Check sheet for the modelled part. Datum: model origin and axes. Units: mm. Coordinates: 2 decimals unless noted, no trailing zeros. Loops run counter-clockwise (first coordinate to the right, second up) from the corner with the lowest first, then second, coordinate; pieces in that order, holes last. Notation, with made-up numbers: (21, 77) - (32, 77) arc R23 ccw to (32, 87) - close; hole circle Ø11 at (12, 67.5). An arc over 180 degrees is marked (long way). Use a Markdown table: item, result. Add a question column.
1) Go/stop test with flat-tipped pins: P1, Ø3, axis at x = 56.5, z = -72.5, coming from the -Y side; P2, Ø9.5, axis at x = -42.43, z = 42.43, coming from the -Y side; P3, Ø3.5, axis at x = -56.5, z = -57.5, coming from the +Y side. Record where each tip stops, or that it passes through.
2) Thickness scan on line 1 (Z direction, x = -72.5, y = 0.25); line 2 (X direction, y = 0.35, z = 72.5); line 3 (Z direction, x = -42.5, y = 0.95). Record the ranges inside material, lowest first.
3) Sectioned sample at A-A, the plane x = -12. Enter the section's corners in (y, z).
4) Sectioned sample at B-B, the plane y = 2.3. State how many separate pieces and enclosed holes the cut face has, then the cut area to 3 significant figures.
5) Sectioned sample at C-C, the plane x = 44.5. Enter the section's corners in (y, z), then the cut area to 3 significant figures.
6) Draft check along Z on faces 1 (the cylindrical face through (-55.984, 1.479, -0.527)), 2 (the flat face through (-1, 0, -1)). Enter one of: pulls with the +Z half, pulls with the -Z half, needs draft (parallel to the pull), parting line crosses it, or undercut.
from build123d import *

# Parameters (mm, degrees)
SKETCH_1_W      = 155
SKETCH_1_H      = 154
SKETCH_1_R      = 1.55
SKETCH_1_R_2    = 2.05
SKETCH_1_R_3    = 4.05
EXTRUDE_1_DEPTH = 3
FILLET_1_R      = 1.5
CHAMFER_1_SIZE  = 1.5
CHAMFER_1_SIZE2 = 2.598076211


with BuildPart() as part:
    # 草图1 → 凸台-拉伸1 (new body)
    with BuildSketch(Plane(origin=(0, 0, 0), x_dir=(1, 0, 0), z_dir=(0, 1, 0))):
        Rectangle(SKETCH_1_W, SKETCH_1_H)
        with Locations(Location((56.5, 72.5, 0), (0, 0, 270))):
            Circle(SKETCH_1_R, mode=Mode.SUBTRACT)
        with Locations(Location((72.5, 72.5, 0), (0, 0, 270))):
            Circle(SKETCH_1_R, mode=Mode.SUBTRACT)
        with Locations(Location((72.5, 57.5, 0), (0, 0, 90))):
            Circle(SKETCH_1_R, mode=Mode.SUBTRACT)
        with Locations(Location((56.5, 57.5, 0), (0, 0, 90))):
            Circle(SKETCH_1_R, mode=Mode.SUBTRACT)
        with Locations(Location((-56.5, 57.5, 0), (0, 0, 270))):
            Circle(SKETCH_1_R, mode=Mode.SUBTRACT)
        with Locations(Location((-72.5, 57.5, 0), (0, 0, 270))):
            Circle(SKETCH_1_R, mode=Mode.SUBTRACT)
        with Locations(Location((-72.5, 72.5, 0), (0, 0, 90))):
            Circle(SKETCH_1_R, mode=Mode.SUBTRACT)
        with Locations(Location((-56.5, 72.5, 0), (0, 0, 90))):
            Circle(SKETCH_1_R, mode=Mode.SUBTRACT)
        with Locations(Location((56.5, -57.5, 0), (0, 0, 270))):
            Circle(SKETCH_1_R, mode=Mode.SUBTRACT)
        with Locations(Location((72.5, -57.5, 0), (0, 0, 270))):
            Circle(SKETCH_1_R, mode=Mode.SUBTRACT)
        with Locations(Location((72.5, -72.5, 0), (0, 0, 90))):
            Circle(SKETCH_1_R, mode=Mode.SUBTRACT)
        with Locations(Location((56.5, -72.5, 0), (0, 0, 90))):
            Circle(SKETCH_1_R, mode=Mode.SUBTRACT)
        with Locations(Location((-56.5, -57.5, 0), (0, 0, 90))):
            Circle(SKETCH_1_R, mode=Mode.SUBTRACT)
        with Locations(Location((-72.5, -57.5, 0), (0, 0, 90))):
            Circle(SKETCH_1_R, mode=Mode.SUBTRACT)
        with Locations(Location((-56.5, -72.5, 0), (0, 0, 270))):
            Circle(SKETCH_1_R, mode=Mode.SUBTRACT)
        with Locations(Location((-72.5, -72.5, 0), (0, 0, 270))):
            Circle(SKETCH_1_R, mode=Mode.SUBTRACT)
        with Locations(Location((-12, 17.5, 0), (0, 0, 270))):
            Circle(SKETCH_1_R_2, mode=Mode.SUBTRACT)
        with Locations(Location((12, 17.5, 0), (0, 0, 270))):
            Circle(SKETCH_1_R_2, mode=Mode.SUBTRACT)
        with Locations(Location((12, -17.5, 0), (0, 0, 90))):
            Circle(SKETCH_1_R_2, mode=Mode.SUBTRACT)
        with Locations(Location((-12, -17.5, 0), (0, 0, 90))):
            Circle(SKETCH_1_R_2, mode=Mode.SUBTRACT)
        with Locations(Location((60, 0, 0), (0, 0, 270))):
            Circle(SKETCH_1_R_3, mode=Mode.SUBTRACT)
        with Locations(Location((42.426406871, -42.426406871, 0), (0, 0, 270))):
            Circle(SKETCH_1_R_3, mode=Mode.SUBTRACT)
        with Locations(Location((0, -60, 0), (0, 0, 270))):
            Circle(SKETCH_1_R_3, mode=Mode.SUBTRACT)
        with Locations(Location((-42.426406871, -42.426406871, 0), (0, 0, 270))):
            Circle(SKETCH_1_R_3, mode=Mode.SUBTRACT)
        with Locations(Location((-60, 0, 0), (0, 0, 270))):
            Circle(SKETCH_1_R_3, mode=Mode.SUBTRACT)
        with Locations(Location((-42.426406871, 42.426406871, 0), (0, 0, 270))):
            Circle(SKETCH_1_R_3, mode=Mode.SUBTRACT)
        with Locations(Location((0, 60, 0), (0, 0, 270))):
            Circle(SKETCH_1_R_3, mode=Mode.SUBTRACT)
        with Locations(Location((42.426406871, 42.426406871, 0), (0, 0, 270))):
            Circle(SKETCH_1_R_3, mode=Mode.SUBTRACT)
    extrude(amount=EXTRUDE_1_DEPTH)

    # 圆角1
    fillet_1_edges = [part.edges().sort_by_distance(p)[0] for p in [
        (-77.5, 1.5, -77),
        (77.5, 1.5, -77),
        (77.5, 1.5, 77),
        (-77.5, 1.5, 77),
    ]]
    fillet(fillet_1_edges, radius=FILLET_1_R)

    # 倒角1
    chamfer_1_edges = [part.edges().sort_by_distance(p)[0] for p in [
        (72.5, 3, -74.05),
        (72.5, 3, -55.95),
        (56.5, 3, -74.05),
        (56.5, 3, -55.95),
        (-56.5, 3, -59.05),
        (-72.5, 3, -59.05),
        (-72.5, 3, -70.95),
        (-56.5, 3, -70.95),
        (56.5, 3, 55.95),
        (72.5, 3, 55.95),
        (72.5, 3, 74.05),
        (56.5, 3, 74.05),
        (-56.5, 3, 59.05),
        (-72.5, 3, 59.05),
        (-56.5, 3, 70.95),
        (-72.5, 3, 70.95),
    ]]
    chamfer_1_side = [part.faces().sort_by_distance(p)[0] for p in [
        (0, 3, 0),
    ]]
    chamfer(chamfer_1_edges, length=CHAMFER_1_SIZE, length2=CHAMFER_1_SIZE2, reference=chamfer_1_side[0])


solid = part.part
Solved:
| question | item | result |
|---|---|---|
| 1 | P1 | passes through |
| 1 | P2 | stops at y = 0 |
| 1 | P3 | stops at y = 0.75 |
| 2 | line 1 | z = -77 to -74.05, -70.95 to -59.05, -55.95 to 55.95, 59.05 to 70.95, 74.05 to 77 |
| 2 | line 2 | x = -77.5 to -74.05, -70.95 to -58.05, -54.95 to 54.95, 58.05 to 70.95, 74.05 to 77.5 |
| 2 | line 3 | z = -77 to -46.48, -38.38 to 38.38, 46.48 to 77 |
| 3 | outline | (0, -77) - (3, -77) - (3, -19.55) - (0, -19.55) - close; (0, -15.45) - (3, -15.45) - (3, 15.45) - (0, 15.45) - close; (0, 19.55) - (3, 19.55) - (3, 77) - (0, 77) - close |
| 4 | separate pieces | 1 |
| 4 | enclosed holes | 28 |
| 4 | area | 23,100 mm2 |
| 5 | outline | (0, -77) - (3, -77) - (3, -45.91) - (0, -45.91) - close; (0, -38.95) - (3, -38.95) - (3, 38.95) - (0, 38.95) - close; (0, 45.91) - (3, 45.91) - (3, 77) - (0, 77) - close |
| 5 | area | 420 mm2 |
| 6 | face 1 | undercut |
| 6 | face 2 | needs draft |
